The listing builds one solid part. Answer for the finished solid, in the listing's coordinates (mm). A direction names the side the tool comes from. Coordinates: 2 decimals unless noted, no trailing zeros. Loops run counter-clockwise (first coordinate to the right, second up) from the corner with the lowest first, then second, coordinate; pieces in that order, holes last. Notation, with made-up numbers: M 61.25,34.5 L 117.25,34.5 A34 ccw 117.25,66.5 Z; hole C 60.5,-2 d8. An arc over 180 degrees is marked long. Answer as a JSON object with one key per item and string values. Group by question number.
1. A cutting plane is placed at B-B on z = 2.65. Give the vertices of the cut face in (x, y), and give its area (3 significant figures).
2. Given pin 1 (2.5 mm diameter, centred on x = -33.5, z = 1.5, fed in from -Y), flat-ended and moving along its own axis, determine where the tip first touches the part or whether it passes through.
3. Determine the mould class of faces 1 (the face through (-65, -18, 3)), 2 (the face through (40, -37.5, 2)), 3 (the face through (-15, -43, 3)), 4 (the face through (65, -18, 3)) for opening direction X: released by +X, released by -X, zero draft, split by the parting line, or undercut.
4. A cutting plane is placed at A-A on y = -44. Give the vertices of the cut face in (x, z).
5. For faces 5 (the face through (-55, -43, 3)), 6 (the face through (20, -47.5, 3)), determine the directions among +Z, -Z, +X, -X, +Y, -Y from which every point of the face is accessible in a straight line to the end or side of a thin tool.
6. Straight lines are drawn through the part: L1, parallel to X at y = -43.5, z = 2.95; L2, parallel to Y at x = -13, z = 4.5. For each, find the intervals that lie inside material, in ascending order.
7. A cutting plane is placed at C-C on x = -6. Give the vertices of the cut face in (y, z), and give its area (3 significant figures).
from build123d import *

# Parameters (mm, degrees)
ESQUISSE1_W                = 130
ESQUISSE1_H                = 50
BOSS_EXTRU_1_DEPTH         = 5
ESQUISSE2_W                = 10
ESQUISSE2_H                = 10
BOSS_EXTRU_2_DEPTH         = 5
R_P_TITION_LIN_AIRE1_COUNT = 4
R_P_TITION_LIN_AIRE1_PITCH = 40


with BuildPart() as part:
    # Esquisse1 → Boss.-Extru.1 (new body)
    with BuildSketch(Plane.XY):
        with Locations((0, -12.5)):
            Rectangle(ESQUISSE1_W, ESQUISSE1_H)
    extrude(amount=BOSS_EXTRU_1_DEPTH)

    # Esquisse2 → Boss.-Extru.2 (add)
    with BuildSketch(Plane.XY.offset(5)):
        with Locations((-60, -42.5)):
            Rectangle(ESQUISSE2_W, ESQUISSE2_H)
    boss_extru_2 = extrude(amount=-BOSS_EXTRU_2_DEPTH)

    # Répétition linéaire1: Boss.-Extru.2 ×4
    with Locations(*[(i * R_P_TITION_LIN_AIRE1_PITCH, 0, 0) for i in range(1, R_P_TITION_LIN_AIRE1_COUNT)]):
        add(boss_extru_2)


solid = part.part
From the geometry:
{
 "1": {"outline": "M -65,-47.5 L -55,-47.5 L -55,-37.5 L -25,-37.5 L -25,-47.5 L -15,-47.5 L -15,-37.5 L 15,-37.5 L 15,-47.5 L 25,-47.5 L 25,-37.5 L 55,-37.5 L 55,-47.5 L 65,-47.5 L 65,12.5 L -65,12.5 Z", "area": "6,900 mm²"},
 "2": {"pin 1": "stops at y = -37.5"},
 "3": {"face 1": "released by -X", "face 2": "undercut", "face 3": "undercut", "face 4": "released by +X"},
 "4": {"outline": "M -65,0 L -55,0 L -55,5 L -65,5 Z; M -25,0 L -15,0 L -15,5 L -25,5 Z; M 15,0 L 25,0 L 25,5 L 15,5 Z; M 55,0 L 65,0 L 65,5 L 55,5 Z"},
 "5": {"face 5": "+Z, -Z, -Y", "face 6": "+Z, -Z, +X, -X, -Y"},
 "6": {"L1": "x = -65 to -55, -25 to -15, 15 to 25, 55 to 65", "L2": "y = -37.5 to 12.5"},
 "7": {"outline": "M -37.5,0 L 12.5,0 L 12.5,5 L -37.5,5 Z", "area": "250 mm²"}
}
